For this review, take the finished solid that the model builds, in its own axes (mm). A direction names the side the tool comes from. Coordinates: 2 decimals unless noted, no trailing zeros. Write each loop counter-clockwise with the first axis right and the second up, starting at its lowest first coordinate (ties: lowest second). Pieces come first, ordered by that corner, then holes. Notation, with made-up numbers: M 70,-3.75 L 99,-3.75 A22 ccw 99,13.25 Z; hole C -30,-31.75 d7. An arc over 180 degrees is marked long. One line per question, with ' | ' between items.
from build123d import *

# Parameters (mm, degrees)
F0_R     = 1.75
F1_DEPTH = 3


with BuildPart() as f1:
    # F0 (on Top) → F1 (new body)
    with BuildSketch(Plane.XY):
        with BuildLine():
            Line((80, 4), (3, 4))
            ThreePointArc((3, 4), (-5, 0), (3, -4))
            Line((3, -4), (80, -4))
            ThreePointArc((80, -4), (76, 0), (80, 4))
        make_face()
        Circle(F0_R, mode=Mode.SUBTRACT)
        with BuildLine():
            ThreePointArc((84, 0), (82.828427, 2.828427), (80, 4))
            ThreePointArc((80, 4), (76, 0), (80, -4))
            ThreePointArc((80, -4), (82.828427, -2.828427), (84, 0))
        make_face()
    extrude(amount=F1_DEPTH)


solid = f1.part
1. Take a section at B-B on y = 1. State the section outline as (x, z) points, plus the area to 3 significant figures.
Computed values:
outline: M -4.9,0 L -1.44,0 L -1.44,3 L -4.9,3 Z; M 1.44,0 L 83.87,0 L 83.87,3 L 1.44,3 Z | area: 258 mm2
2. Clearance check with a flat-ended pin moving along its axis: P1, Ø1.5, axis at x = 28, z = 1.5, coming from the -Y side. State where the tip first meets the part, or that it passes through.
Computed values:
P1: stops at y = -4
3. For line 1 along Y through (x, z) = (0, 1.35); line 2 along Y through (x, z) = (43, 1.45); line 3 along X through (y, z) = (-1.5, 1.05), list the stretches that pass through material, from the lowest coordinate up.
Computed values:
line 1: y = -5 to -1.75, 1.75 to 5 | line 2: y = -4 to 4 | line 3: x = -4.77 to -0.9, 0.9 to 83.71
4. Take a section at D-D on x = 46.5. State the section outline as (y, z) points, plus the area to 3 significant figures.
Computed values:
outline: M -4,0 L 4,0 L 4,3 L -4,3 Z | area: 24.0 mm2
5. Machinability: for faces 4 (the flat face through (41, -4, 1)), 5 (the flat face through (42, 4, 1)), 6 (the flat face through (39, 0, 0)), which of the approach directions +Z, -Z, +X, -X, +Y, -Y give a long, thin tool a straight path to every point of the face, cutting with its end or side? Answer none if there is none.
Computed values:
face 4: +Z, -Z, +X, -Y | face 5: +Z, -Z, +X, +Y | face 6: -Z, +X, -X, +Y, -Y
6. Take a section at A-A on x = 0. State the section outline as (y, z) points.
Computed values:
outline: M -5,0 L -1.75,0 L -1.75,3 L -5,3 Z; M 1.75,0 L 5,0 L 5,3 L 1.75,3 Z
7. Draft analysis for pull direction Y (two halves, no side actions). For faces 1 (the cylindrical face through (1.617, -0.67, 1.479)), 2 (the cylindrical face through (-5, 0, 1)), 3 (the flat face through (39, 0, 3)), state which applies: pulls with the +Y half, pulls with the -Y half, needs draft (parallel to the pull), parting line crosses it, or undercut.
Computed values:
face 1: undercut | face 2: parting line crosses it | face 3: needs draft
8. Take a section at C-C on z = 1.6. State the section outline as (x, y) points.
Computed values:
outline: M 3,-4 L 80,-4 A4 ccw 80,4 L 3,4 A5 ccw long Z; hole C 0,0 d3.5
